Can you work these out from the drawing? Everything is in mm from the part's minimum corner. A direction names the side the tool comes from. Round coordinates to 2 decimals unless told otherwise and drop trailing zeros. Write each loop counter-clockwise with the first axis right and the second up, starting at its lowest first coordinate (ties: lowest second). Pieces come first, ordered by that corner, then holes.
Q1. For the marked faces 1, 2 and 3, which set-ups out of +Z, -Z, +X, -X, +Y, -Y let a thin tool reach every point of the face, with its end or its side?
Q2. If we section it at B-B (y = 18): Please give me the cut outline in (x, z), plus the area to 3 significant figures.
Q3. Please list where these lines run through material, in increasing order: line 1 along X through (y, z) = (30.5, 2.75); line 2 along Y through (x, z) = (63.5, 4.75); line 3 along Z through (x, y) = (31.5, 75.5).
Q4. I'm going to push flat-ended pins straight in: pin 1 Ø4 at (x, y) = (23, 15) entering from -Z; pin 2 Ø2 at (x, z) = (56.5, 4.5) entering from +Y; pin 3 Ø5 at (x, z) = (60.5, 4.5) entering from -Y. Where does each tip first touch, or does it pass through?
Q5. If we section it at A-A (z = 18.75): Give the number of separate pieces and of enclosed holes in the cut face, plus the area to 3 significant figures.
Q6. We'd pull the mould along Y, two halves only. Please class the marked faces 4, 5 and 6: +Y half, -Y half, draft (parallel to the pull), parting line (faces both ways), or undercut.
Q7. If we section it at D-D (x = 72): Please give me the cut outline in (y, z).
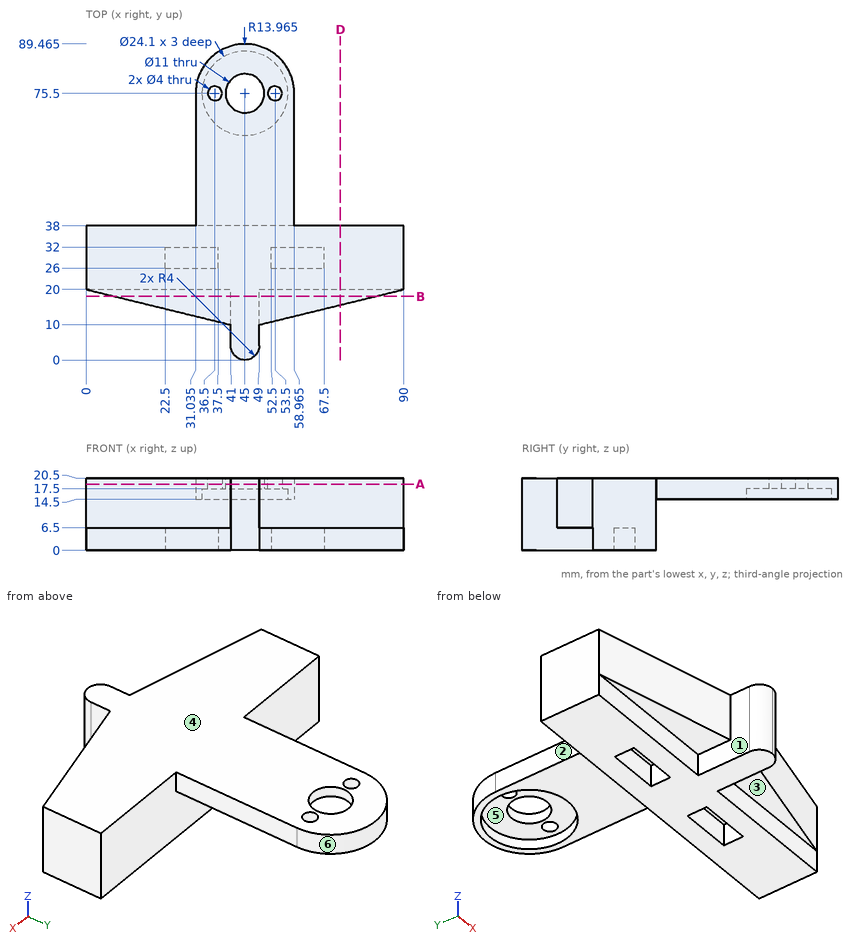
A:
1. face 1: -Z, -X, -Y
1. face 2: +Z, -Z, -X, +Y
1. face 3: -Z, +X, -Y
2. outline: (8.2, 6.5) - (41, 6.5) - (41, 0) - (49, 0) - (49, 6.5) - (81.8, 6.5) - (81.8, 20.5) - (8.2, 20.5) - close
2. area: 1,080 mm2
3. line 1: x = 0 to 22.5, 37.5 to 52.5, 67.5 to 90
3. line 2: y = 20 to 26, 32 to 38
3. line 3: z = 14.5 to 20.5
4. pin 1: stops at z = 6.5
4. pin 2: stops at y = 38
4. pin 3: stops at y = 12.44
5. separate pieces: 1
5. enclosed holes: 3
5. area: 3,420 mm2
6. face 4: draft
6. face 5: undercut
6. face 6: +Y half
7. outline: (15.61, 6.5) - (20, 6.5) - (20, 0) - (38, 0) - (38, 20.5) - (15.61, 20.5) - close
